Design review of the part built by this model. Coordinates are the model's own, in mm. Face numbers are marked on the shaded views. Coordinates: 2 decimals unless noted, no trailing zeros. Write each loop counter-clockwise with the first axis right and the second up, starting at its lowest first coordinate (ties: lowest second). Pieces come first, ordered by that corner, then holes.
Q1. Mouldability with a two-part tool opening along Y and no side actions: class the marked faces 1, 2, 3 and 4 as pulls with the +Y half, pulls with the -Y half, needs draft (parallel to the pull), parting line crosses it, or undercut.
Q2. Take a section at A-A (z = 8). Give the boundary of the cut face in (x, y).
Q3. Insertion check: pin 1 (4.5 mm diameter, centred on x = 204.5, y = 10, fed in from +Z); pin 2 (4 mm diameter, centred on x = 27, y = 8, fed in from -Z); pin 3 (1.6 mm diameter, centred on x = 7.5, y = 33, fed in from +Z). Each pin has a flat end and moves straight along its axis. Give the tip position at first contact, or say it passes through.
Q4. Take a section at C-C (x = 138). Give the boundary of the cut face in (y, z).
Q5. For probe 1 along X at (y, z) = (24, 0.5); probe 2 along Y at (x, z) = (87, 12); probe 3 along Y at (x, z) = (122, 1), list the stretches that pass through material, from the lowest coordinate up.
Q6. Take a section at D-D (x = 198.5). Give the boundary of the cut face in (y, z).
Q7. Take a section at B-B (y = 27). Give the boundary of the cut face in (x, z), and give its area (3 significant figures).
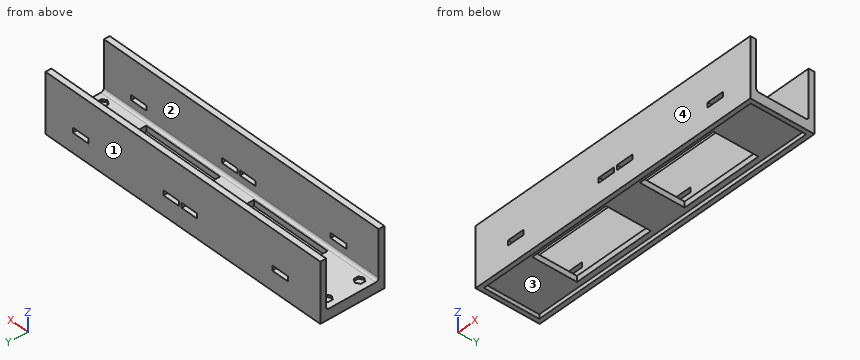
```python
from build123d import *

# Parameters (mm, degrees)
FACEPLATESKETCH_W      = 212
FACEPLATESKETCH_H      = 44.45
FACEPLATEPAD_DEPTH     = 4
BOTTOMWALLSKETCH_W     = 212
BOTTOMWALLSKETCH_H     = 4
BOTTOMWALLPAD_DEPTH    = 34
TOPWALLSKETCH_W        = 212
TOPWALLSKETCH_H        = 4
TOPWALLPAD_DEPTH       = 34
LIPBLOCKSKETCH_W       = 212
LIPBLOCKSKETCH_H       = 44.45
LIPBLOCKPAD_DEPTH      = 3
LIPPOCKETSKETCH_W      = 206
LIPPOCKETSKETCH_H      = 38.45
LIPPOCKET_DEPTH        = 3
JOINTHOLESSKETCH_R     = 1.6
JOINTHOLESPOCKET_DEPTH = 3.001
NUTRECESSPOCKET_DEPTH  = 1.5
BOXCUTOUTSKETCH_W      = 57
BOXCUTOUTSKETCH_H      = 31
BOXCUTOUTPOCKET_DEPTH  = 38.001
WALLFILLETS_R          = 2
TOPSLOTSKETCH_W        = 12
TOPSLOTSKETCH_H        = 3.4
TOPSLOTPOCKET_DEPTH    = 44.451


with BuildPart() as part:
    # FacePlateSketch → FacePlatePad (new body)
    with BuildSketch(Plane.XY):
        with Locations((106, 22.225)):
            Rectangle(FACEPLATESKETCH_W, FACEPLATESKETCH_H)
    extrude(amount=FACEPLATEPAD_DEPTH)

    # BottomWallSketch (on Face6 of FacePlatePad) → BottomWallPad (join)
    with BuildSketch(Plane.XY.offset(4)):
        with Locations((106, 2)):
            Rectangle(BOTTOMWALLSKETCH_W, BOTTOMWALLSKETCH_H)
    extrude(amount=BOTTOMWALLPAD_DEPTH)

    # TopWallSketch (on Face6 of FacePlatePad) → TopWallPad (join)
    with BuildSketch(Plane.XY.offset(4)):
        with Locations((106, 42.45)):
            Rectangle(TOPWALLSKETCH_W, TOPWALLSKETCH_H)
    extrude(amount=TOPWALLPAD_DEPTH)

    # LipBlockSketch → LipBlockPad (join)
    with BuildSketch(Plane.XY):
        with Locations((106, 22.225)):
            Rectangle(LIPBLOCKSKETCH_W, LIPBLOCKSKETCH_H)
    extrude(amount=-LIPBLOCKPAD_DEPTH)

    # LipPocketSketch → LipPocket (cut)
    with BuildSketch(Plane.XY):
        with Locations((106, 22.225)):
            Rectangle(LIPPOCKETSKETCH_W, LIPPOCKETSKETCH_H)
    extrude(amount=-LIPPOCKET_DEPTH, mode=Mode.SUBTRACT)

    # JointHolesSketch → JointHolesPocket (cut, through all)
    with BuildSketch(Plane.XY):
        with Locations((7, 11)):
            Circle(JOINTHOLESSKETCH_R)
        with Locations((205, 11)):
            Circle(JOINTHOLESSKETCH_R)
        with Locations((7, 33.45)):
            Circle(JOINTHOLESSKETCH_R)
        with Locations((205, 33.45)):
            Circle(JOINTHOLESSKETCH_R)
    extrude(amount=-JOINTHOLESPOCKET_DEPTH, mode=Mode.SUBTRACT)

    # NutRecessSketch (on Face6 of FacePlatePad) → NutRecessPocket (cut)
    with BuildSketch(Plane.XY.offset(4)):
        Polygon((9.75, 12.587713), (7, 14.175426), (4.25, 12.587713), (4.25, 9.412287), (7, 7.824574), (9.75, 9.412287), align=None)
        Polygon((207.75, 12.587713), (205, 14.175426), (202.25, 12.587713), (202.25, 9.412287), (205, 7.824574), (207.75, 9.412287), align=None)
        Polygon((9.75, 35.037713), (7, 36.625426), (4.25, 35.037713), (4.25, 31.862287), (7, 30.274574), (9.75, 31.862287), align=None)
        Polygon((207.75, 35.037713), (205, 36.625426), (202.25, 35.037713), (202.25, 31.862287), (205, 30.274574), (207.75, 31.862287), align=None)
    extrude(amount=-NUTRECESSPOCKET_DEPTH, mode=Mode.SUBTRACT)

    # BoxCutoutSketch → BoxCutoutPocket (cut, through all)
    with BuildSketch(Plane.XY):
        with Locations((64.5, 22.5)):
            Rectangle(BOXCUTOUTSKETCH_W, BOXCUTOUTSKETCH_H)
        with Locations((147.5, 22.5)):
            Rectangle(BOXCUTOUTSKETCH_W, BOXCUTOUTSKETCH_H)
    extrude(amount=BOXCUTOUTPOCKET_DEPTH, mode=Mode.SUBTRACT)

    # WallFillets
    wallfillets_edges = [part.edges().sort_by_distance(p)[0] for p in [
        (106, 4, 4),
        (106, 40.45, 4),
    ]]
    fillet(wallfillets_edges, radius=WALLFILLETS_R)

    # TopSlotSketch (on Face10 of WallFillets) → TopSlotPocket (cut, through all)
    with BuildSketch(Plane(origin=(0, 44.45, 0), x_dir=(-1, 0, 0), z_dir=(0, 1, 0))):
        with Locations((-31, 12)):
            Rectangle(TOPSLOTSKETCH_W, TOPSLOTSKETCH_H)
        with Locations((-101, 12)):
            Rectangle(TOPSLOTSKETCH_W, TOPSLOTSKETCH_H)
        with Locations((-115, 12)):
            Rectangle(TOPSLOTSKETCH_W, TOPSLOTSKETCH_H)
        with Locations((-185, 12)):
            Rectangle(TOPSLOTSKETCH_W, TOPSLOTSKETCH_H)
    extrude(amount=-TOPSLOTPOCKET_DEPTH, mode=Mode.SUBTRACT)


solid = part.part
```
Response:
1. face 1: pulls with the +Y half
1. face 2: undercut
1. face 3: undercut
1. face 4: pulls with the -Y half
2. outline: (0, 0) - (212, 0) - (212, 4) - (0, 4) - close; (0, 40.45) - (212, 40.45) - (212, 44.45) - (0, 44.45) - close
3. pin 1: stops at z = 4
3. pin 2: stops at z = 0
3. pin 3: stops at z = 2.5
4. outline: (0, -3) - (3, -3) - (3, 0) - (7, 0) - (7, 4) - (6, 4) arc R2 cw to (4, 6) - (4, 38) - (0, 38) - close; (38, 0) - (41.45, 0) - (41.45, -3) - (44.45, -3) - (44.45, 38) - (40.45, 38) - (40.45, 6) arc R2 cw to (38.45, 4) - (38, 4) - close
5. probe 1: x = 0 to 36, 93 to 119, 176 to 212
5. probe 2: y = 0 to 4, 40.45 to 44.45
5. probe 3: y = 0 to 7, 38 to 44.45
6. outline: (0, -3) - (3, -3) - (3, 0) - (41.45, 0) - (41.45, -3) - (44.45, -3) - (44.45, 38) - (40.45, 38) - (40.45, 6) arc R2 cw to (38.45, 4) - (6, 4) arc R2 cw to (4, 6) - (4, 38) - (0, 38) - close
7. outline: (0, -3) - (3, -3) - (3, 0) - (36, 0) - (36, 4) - (0, 4) - close; (93, 0) - (119, 0) - (119, 4) - (93, 4) - close; (176, 0) - (209, 0) - (209, -3) - (212, -3) - (212, 4) - (176, 4) - close
7. area: 410 mm2
